The figure shows three views and two pictorial views of one solid part (mm, origin at its lowest corner). Answer the questions. Coordinates: 2 decimals unless noted, no trailing zeros. Order: outer loops, then holes, each group sorted by start corner. A loop starts at its lowest first (then second) coordinate and runs counter-clockwise, first axis right, second up. Notation, with made-up numbers: (28.5, 48.5) -> (81.5, 48.5) arc R15 ccw to (81.5, 52.5) -> close; hole circle Ø5 at (15.25, 46). An arc over 180 degrees is marked (long way). Return JSON: item names as keys, results as strings.
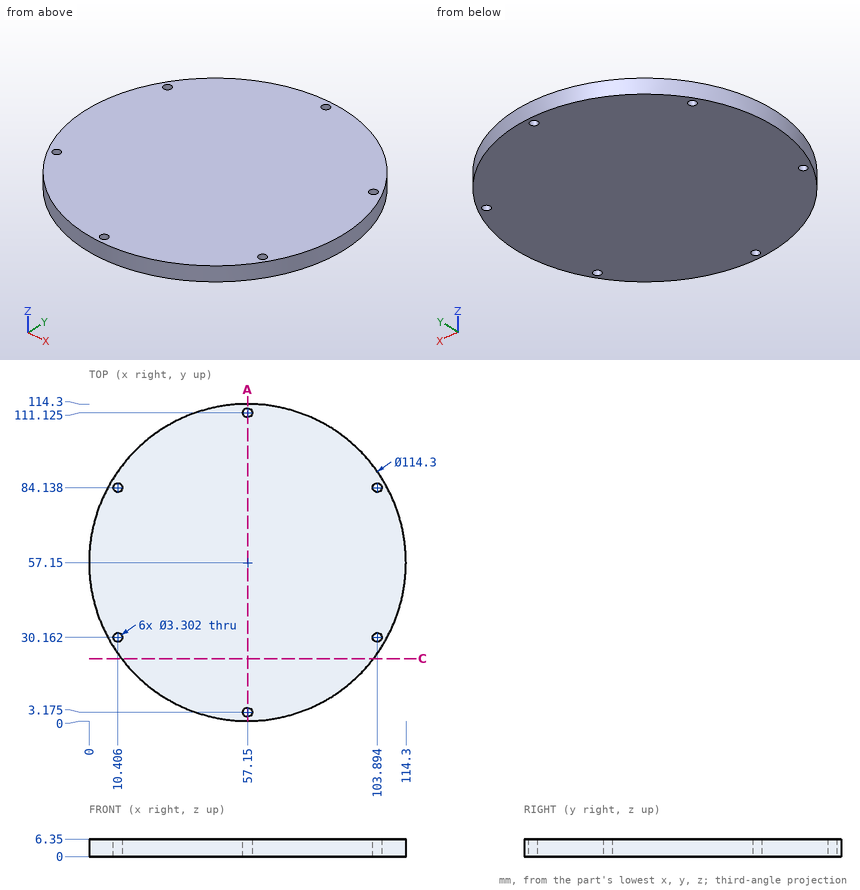
1. The part is cut by section A-A on x = 57.15. Give the number of separate pieces and of enclosed holes in the cut face, and give its area (3 significant figures).
Answer block:
{"separate pieces": "3", "enclosed holes": "0", "area": "684 mm2"}
2. The part is cut by section C-C on y = 22.5. Give the vertices of the cut face in (x, z).
Answer block:
{"outline": "(11.7, 0) -> (102.6, 0) -> (102.6, 6.35) -> (11.7, 6.35) -> close"}
3. Consider line 1 (Y direction, x = 11, z = 5) (1 decimal); line 2 (Y direction, x = 105, z = 5) (1 decimal); line 3 (Y direction, x = 20, z = 5.5). Determine where each line is inside the solid, lowest interval first. Write a range as from..to.
Answer block:
{"line 1": "y = 23.4..28.6, 31.7..82.6, 85.7..90.9", "line 2": "y = 25.9..28.9, 31.4..82.9, 85.4..88.4", "line 3": "y = 13.72..100.58"}
4. Each of these flat-tipped pins is pushed along its axis until it touches: pin 1 Ø1 at (y, z) = (50.5, 3) entering from +X; pin 2 Ø3 at (x, z) = (19, 2) entering from -Y; pin 3 Ø1.5 at (x, z) = (22, 3) entering from +Y. Where does it stop, or does it pass through?
Answer block:
{"pin 1": "stops at x = 113.97", "pin 2": "stops at y = 13.3", "pin 3": "stops at y = 102.79"}
